Work out the finished part from the listing and answer in its coordinate system (mm). Give positions to 0.01 mm unless a question says otherwise; leave off trailing zeros. Loops run counter-clockwise (first coordinate to the right, second up) from the corner with the lowest first, then second, coordinate; pieces in that order, holes last.
Autodesk Inventor part; units mm, degrees
ref_plane "YZ Plane" through (0, 0, 0) normal (1, 0, 0) x (0, 1, 0)
ref_plane "XZ Plane" through (0, 0, 0) normal (0, 1, 0) x (-1, 0, 0)
ref_plane "XY Plane" through (0, 0, 0) normal (0, 0, 1) x (1, 0, 0)
sketch "スケッチ1" plane through (0, 0, 0) normal (0, 0, 1) x (1, 0, 0)
  line L0 (24, 0) -> (24, 100)
  line L1 (0, 100) -> (0, 0)
  line L2 (12, 100) -> (12, 0) construction
  arc A0 (24, 100) -> (0, 100) centre (12, 100) ccw
  arc A1 (0, 0) -> (24, 0) centre (12, 0) ccw
  circle A2 centre (12, 0) radius 3.5
  circle A3 centre (12, 100) radius 3.5
  circle A4 centre (12, 50) radius 5
  dimension "d35" = 24
  dimension "d36" = 100
  dimension "d37" = 7
  dimension "d38" = 7
  dimension "d41" = 10
extrude "押し出し1" add sketch "スケッチ1" along normal blind 2
sketch "スケッチ3" plane through (0, 0, 2) normal (0, 0, 1) x (1, 0, 0)
  circle A0 centre (12, 0) radius 3.5
  circle A1 centre (12, 100) radius 3.5
  circle A2 centre (12, 50) radius 5
  arc A3 (24, 100) -> (0, 100) centre (12, 100) ccw
  line L0 (0, 100) -> (0, 0)
  arc A4 (0, 0) -> (24, 0) centre (12, 0) ccw
  line L1 (24, 0) -> (24, 100)
  line L2 (12, 50) -> (24, 50) construction
  line L3 (24, 0) -> (24, 100)
  point P0 (20.5, 50)
  point P1 (12, 58.5)
  point P2 (3.5, 50)
  point P3 (12, 41.5)
  dimension "d42" = 8.5
  dimension "d45" = 360
hole "穴1" at (20.5, 50, 2) at (12, 58.5, 2) at (3.5, 50, 2) at (12, 41.5, 2) direction (0, 0, -1) diameter 2.8 end through all
properties part number "hip_link_motor" material "GFRP"
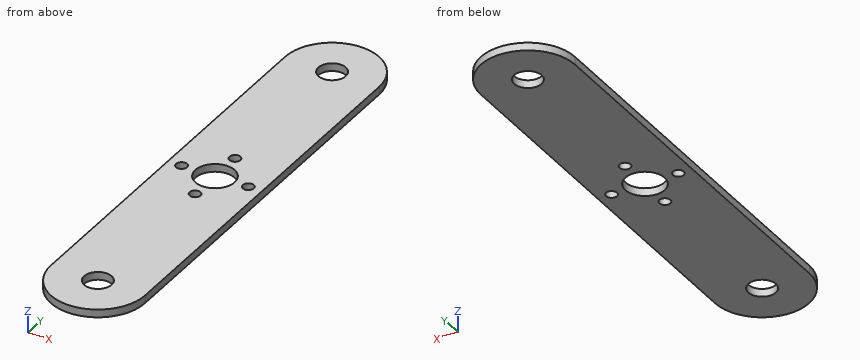
Q1. Section D-D on x = 20.5 is taken. Give the vertices of the cut face in (y, z), plus the area to 3 significant figures.
Q2. Given pin 1 (2.5 mm diameter, centred on x = 20.5, y = 50, fed in from +Z), flat-ended and moving along its own axis, determine where the tip first touches the part or whether it passes through.
Q3. Consider line 1 along Y through (x, z) = (12, 1.25); line 2 along X through (y, z) = (51, 1.55); line 3 along Y through (x, z) = (10.75, 0.9). Determine where each line is inside the solid, lowest interval first.
Q4. Section B-B on z = 1.6 is taken. Give the vertices of the cut face in (x, y).
Q5. Section A-A on y = 58.5 is taken. Give the vertices of the cut face in (x, z), plus the area to 3 significant figures.
Q6. Section C-C on x = 12 is taken. Give the vertices of the cut face in (y, z), plus the area to 3 significant figures.
Check result:
1. outline: (-8.47, 0) - (48.6, 0) - (48.6, 2) - (-8.47, 2) - close; (51.4, 0) - (108.47, 0) - (108.47, 2) - (51.4, 2) - close
1. area: 228 mm2
2. pin 1: passes through
3. line 1: y = -12 to -3.5, 3.5 to 40.1, 42.9 to 45, 55 to 57.1, 59.9 to 96.5, 103.5 to 112
3. line 2: x = 0 to 2.52, 4.48 to 7.1, 16.9 to 19.52, 21.48 to 24
3. line 3: y = -11.93 to -3.27, 3.27 to 40.87, 42.13 to 45.16, 54.84 to 57.87, 59.13 to 96.73, 103.27 to 111.93
4. outline: (0, 0) arc R12 ccw to (24, 0) - (24, 100) arc R12 ccw to (0, 100) - close; hole circle Ø2.8 at (3.5, 50); hole circle Ø10 at (12, 50); hole circle Ø7 at (12, 0); hole circle Ø7 at (12, 100); hole circle Ø2.8 at (12, 41.5); hole circle Ø2.8 at (12, 58.5); hole circle Ø2.8 at (20.5, 50)
5. outline: (0, 0) - (10.6, 0) - (10.6, 2) - (0, 2) - close; (13.4, 0) - (24, 0) - (24, 2) - (13.4, 2) - close
5. area: 42.4 mm2
6. outline: (-12, 0) - (-3.5, 0) - (-3.5, 2) - (-12, 2) - close; (3.5, 0) - (40.1, 0) - (40.1, 2) - (3.5, 2) - close; (42.9, 0) - (45, 0) - (45, 2) - (42.9, 2) - close; (55, 0) - (57.1, 0) - (57.1, 2) - (55, 2) - close; (59.9, 0) - (96.5, 0) - (96.5, 2) - (59.9, 2) - close; (103.5, 0) - (112, 0) - (112, 2) - (103.5, 2) - close
6. area: 189 mm2
